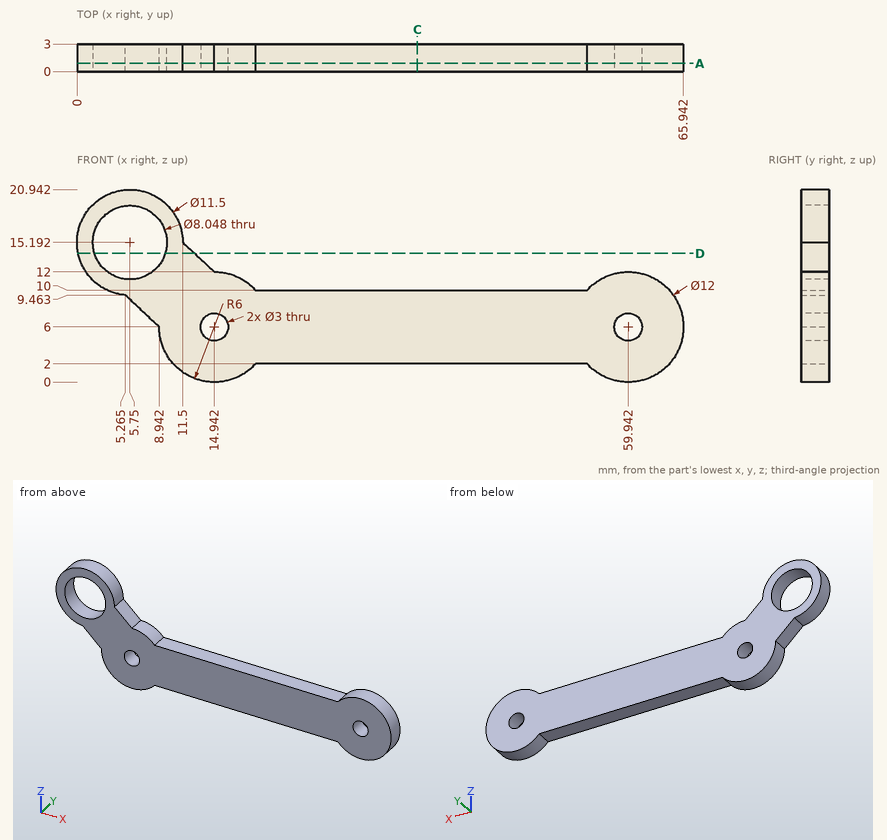
Answer from the drawing. Dimensions are ordinates in mm from the lowest x, y and z of the part. Coordinates: 2 decimals unless noted, no trailing zeros. Order: outer loops, then holes, each group sorted by start corner. A loop starts at its lowest first (then second) coordinate and runs counter-clockwise, first axis right, second up. Notation, with made-up numbers: M -34.75,-2 L -26.75,-2 A17 ccw -26.75,13 Z; hole C 58.5,69.5 d9. An arc over 180 degrees is marked long. Put each result on its own line as item: value. Start each with the question number.
Item 1: Consider probe 1 along Z at (x, y) = (15, 0.65); probe 2 along Z at (x, y) = (44.5, 1); probe 3 along Z at (x, y) = (16, 1.6) (1 decimal). Determine where each line is inside the solid, lowest interval first. Write a range as [from, to].
Item 2: Given pin 1 Ø1.5 at (x, y) = (29.5, 1) entering from +Z; pin 2 Ø0.9 at (x, y) = (31.5, 2) entering from -Z, each flat-ended and moving along its own axis, determine where each tip first touches the part or whether it passes through.
Item 3: Section C-C, the plane x = 37 is taken. Determine the outline of the cut face in (y, z), plus the area to 3 significant figures.
Item 4: Section D-D, the plane z = 14 is taken. Determine the outline of the cut face in (x, y) (1 decimal).
Item 5: Section A-A, the plane y = 0.9 is taken. Count the separate pieces of the cut face and the enclosed holes in it, plus the area to 3 significant figures.
Computed:
1. probe 1: z = [0, 4.5], [7.5, 12]
1. probe 2: z = [2, 10]
1. probe 3: z = [0.1, 4.9], [7.1, 11.9]
2. pin 1: stops at z = 10
2. pin 2: stops at z = 2
3. outline: M 0,2 L 3,2 L 3,10 L 0,10 Z
3. area: 24.0 mm2
4. outline: M 0.1,0 L 1.9,0 L 1.9,3 L 0.1,3 Z; M 9.6,0 L 12.8,0 L 12.8,3 L 9.6,3 Z
5. separate pieces: 1
5. enclosed holes: 3
5. area: 557 mm2
